Check sheet for the modelled part. Datum: model origin and axes. Units: mm. A direction names the side the tool comes from. Coordinates: 2 decimals unless noted, no trailing zeros. Order: outer loops, then holes, each group sorted by start corner. A loop starts at its lowest first (then second) coordinate and runs counter-clockwise, first axis right, second up.
from build123d import *

# Parameters (mm, degrees)
BOSS_EXTRUDE1_DEPTH = 12.7
SKETCH2_W           = 12.7
SKETCH2_H           = 63.5
BOSS_EXTRUDE2_DEPTH = 31.75
SKETCH3_W           = 18
SKETCH3_H           = 3
CUT_EXTRUDE1_DEPTH  = 19.05
SKETCH4_R           = 2
CUT_EXTRUDE2_DEPTH  = 59.973007597
SKETCH5_R           = 2
CUT_EXTRUDE3_DEPTH  = 64.181702256
SKETCH6_W           = 63.5
SKETCH6_H           = 12.7
CUT_EXTRUDE4_DEPTH  = 11.05
SKETCH7_W           = 12.7
SKETCH7_H           = 63.5
CUT_EXTRUDE5_DEPTH  = 11.05
BOSS_EXTRUDE3_START = 3.175
SKETCH8_W           = 33.4
SKETCH8_H           = 63.5
SKETCH8_R           = 2
SKETCH8_W_2         = 6
SKETCH8_H_2         = 18
BOSS_EXTRUDE3_DEPTH = 3.175
SKETCH9_R           = 1.25
SKETCH9_R_2         = 1.5
CUT_EXTRUDE6_DEPTH  = 54.289246101


with BuildPart() as part:
    # Sketch1 → Boss-Extrude1 (new body)
    with BuildSketch(Plane(origin=(0, 0, 0), x_dir=(1, 0, 0), z_dir=(0, 1, 0))):
        Polygon((-22.225, 31.75), (-22.225, -31.75), (0, -31.75), (0, -24.875), (-3, -24.875), (-3, -6.875), (0, -6.875), (0, 0), (0, 6.875), (-3, 6.875), (-3, 24.875), (0, 24.875), (0, 31.75), align=None)
        Polygon((0, -24.875), (0, -31.75), (22.225, -31.75), (22.225, 31.75), (0, 31.75), (0, 24.875), (3, 24.875), (3, 6.875), (0, 6.875), (0, 0), (0, -6.875), (3, -6.875), (3, -24.875), align=None)
    extrude(amount=BOSS_EXTRUDE1_DEPTH)

    # Sketch2 → Boss-Extrude2 (add)
    with BuildSketch(Plane.XZ):
        with Locations((-15.875, 0)):
            Rectangle(SKETCH2_W, SKETCH2_H)
    extrude(amount=BOSS_EXTRUDE2_DEPTH)

    # Sketch3 → Cut-Extrude1 (cut)
    with BuildSketch(Plane.ZY.offset(22.225)):
        with Locations((-15.875, -8.025)):
            Rectangle(SKETCH3_W, SKETCH3_H)
        with Locations((-15.875, -11.025)):
            Rectangle(SKETCH3_W, SKETCH3_H)
        with Locations((15.875, -8.025)):
            Rectangle(SKETCH3_W, SKETCH3_H)
        with Locations((15.875, -11.025)):
            Rectangle(SKETCH3_W, SKETCH3_H)
    extrude(amount=-CUT_EXTRUDE1_DEPTH, mode=Mode.SUBTRACT)

    # Sketch4 → Cut-Extrude2 (cut, through all)
    with BuildSketch(Plane(origin=(0, 12.7, 0), x_dir=(1, 0, 0), z_dir=(0, 1, 0))):
        with Locations(Location((-15.875, 15.875, 0), (0, 0, 270))):
            Circle(SKETCH4_R)
        with Locations(Location((-15.875, -15.875, 0), (0, 0, 270))):
            Circle(SKETCH4_R)
    extrude(amount=-CUT_EXTRUDE2_DEPTH, mode=Mode.SUBTRACT)

    # Sketch5 → Cut-Extrude3 (cut, through all)
    with BuildSketch(Plane.ZY.offset(22.225)):
        with Locations((-15.875, 6.35)):
            Circle(SKETCH5_R)
        with Locations((15.875, 6.35)):
            Circle(SKETCH5_R)
    extrude(amount=-CUT_EXTRUDE3_DEPTH, mode=Mode.SUBTRACT)

    # Sketch6 → Cut-Extrude4 (cut)
    with BuildSketch(Plane(origin=(22.225, 0, 0), x_dir=(0, 0, -1), z_dir=(1, 0, 0))):
        with Locations((0, 6.35)):
            Rectangle(SKETCH6_W, SKETCH6_H)
    extrude(amount=-CUT_EXTRUDE4_DEPTH, mode=Mode.SUBTRACT)

    # Sketch7 → Cut-Extrude5 (cut)
    with BuildSketch(Plane.XZ.offset(31.75)):
        with Locations((-15.875, 0)):
            Rectangle(SKETCH7_W, SKETCH7_H)
    extrude(amount=-CUT_EXTRUDE5_DEPTH, mode=Mode.SUBTRACT)

    # Sketch8 → Boss-Extrude3 (add)
    with BuildSketch(Plane(origin=(0, 12.7, 0), x_dir=(1, 0, 0), z_dir=(0, 1, 0)).offset(BOSS_EXTRUDE3_START)):
        with Locations((-5.525, 0)):
            Rectangle(SKETCH8_W, SKETCH8_H)
        with Locations(Location((-15.875, 15.875, 0), (0, 0, 90))):
            Circle(SKETCH8_R, mode=Mode.SUBTRACT)
        with Locations(Location((-15.875, -15.875, 0), (0, 0, 90))):
            Circle(SKETCH8_R, mode=Mode.SUBTRACT)
        with Locations((0, -15.875)):
            Rectangle(SKETCH8_W_2, SKETCH8_H_2, mode=Mode.SUBTRACT)
        with Locations((0, 15.875)):
            Rectangle(SKETCH8_W_2, SKETCH8_H_2, mode=Mode.SUBTRACT)
    extrude(amount=-BOSS_EXTRUDE3_DEPTH)

    # Sketch9 → Cut-Extrude6 (cut, through all)
    with BuildSketch(Plane(origin=(0, 15.875, 0), x_dir=(1, 0, 0), z_dir=(0, 1, 0))):
        with Locations(Location((-15.875, 26.75, 0), (0, 0, 270))):
            Circle(SKETCH9_R)
        with Locations(Location((-15.875, -26.75, 0), (0, 0, 270))):
            Circle(SKETCH9_R)
        with Locations(Location((-15.875, 0, 0), (0, 0, 270))):
            Circle(SKETCH9_R_2)
    extrude(amount=-CUT_EXTRUDE6_DEPTH, mode=Mode.SUBTRACT)


solid = part.part
(1) Release check for a two-part mould opening along Z. For faces 4 (the flat face through (-16, -12.525, 13.7)), 5 (the flat face through (-22.225, -2, 0)), 6 (the flat face through (-9, 2, -31.75)) record: +Z half, -Z half, draft (parallel to the pull), parting line (faces both ways), or undercut.
Filled in:
face 4: undercut
face 5: draft
face 6: -Z half
(2) Tool access check on faces 1 (the flat face through (3, 10, 16)), 2 (the flat face through (-9.525, -10, 0)), 3 (the flat face through (-16, -10, 24.875)). Record the directions out of +Z, -Z, +X, -X, +Y, -Y that give a thin tool (end or side, any length) a straight path to the whole face; none if there is none.
Filled in:
face 1: +Y, -Y
face 2: +Z, -Z, +X, -Y
face 3: +X, -X
(3) Cross-section at B-B (x = -1). Enter the section's corners in (y, z) (3 decimals).
Filled in:
outline: (0, -31.75) - (15.875, -31.75) - (15.875, -24.875) - (0, -24.875) - close; (0, -6.875) - (15.875, -6.875) - (15.875, 6.875) - (0, 6.875) - close; (0, 24.875) - (15.875, 24.875) - (15.875, 31.75) - (0, 31.75) - close
(4) Cross-section at A-A (z = 0). Enter the section's corners in (x, y) (3 decimals).
Filled in:
outline: (-22.225, -20.7) - (-17.375, -20.7) - (-17.375, 15.875) - (-22.225, 15.875) - close; (-14.375, -20.7) - (-9.525, -20.7) - (-9.525, 0) - (11.175, 0) - (11.175, 15.875) - (-14.375, 15.875) - close
(5) Go/stop test with flat-tipped pins: P1, Ø8, axis at x = 4, z = -19.5, coming from the -Y side; P2, Ø2.5, axis at x = -15.875, z = 15.875, coming from the -Y side. Record where each tip stops, or that it passes through.
Filled in:
P1: stops at y = 0
P2: passes through
(6) Cross-section at C-C (y = 3.5). Enter the section's corners in (x, z) (3 decimals).
Filled in:
outline: (-22.225, -31.75) - (11.175, -31.75) - (11.175, 31.75) - (-22.225, 31.75) - close; hole circle Ø4 at (-15.875, -15.875); hole circle Ø4 at (-15.875, 15.875); hole circle Ø3 at (-15.875, 0); hole circle Ø2.5 at (-15.875, -26.75); hole circle Ø2.5 at (-15.875, 26.75); hole (-3, -24.875) - (3, -24.875) - (3, -6.875) - (-3, -6.875) - close; hole (-3, 6.875) - (3, 6.875) - (3, 24.875) - (-3, 24.875) - close
(7) Cross-section at D-D (x = 5). Enter the section's corners in (y, z) (3 decimals).
Filled in:
outline: (0, -31.75) - (15.875, -31.75) - (15.875, 31.75) - (0, 31.75) - close; hole circle Ø4 at (6.35, -15.875); hole circle Ø4 at (6.35, 15.875)
(8) Thickness scan on probe 1 along Z at (x, y) = (0, 4) (3 decimals); probe 2 along Y at (x, z) = (-15, 22) (3 decimals); probe 3 along Y at (x, z) = (-12.5, -17.5) (3 decimals). Record the ranges inside material, lowest first.
Filled in:
probe 1: z = -31.75 to -24.875, -6.875 to 6.875, 24.875 to 31.75
probe 2: y = -20.7 to -12.525, -6.525 to 15.875
probe 3: y = -20.7 to -12.525, -6.525 to 5.184, 7.516 to 15.875
